Read the model definition and answer for the solid it produces. Units are mm, in the model's axes. A direction names the side the tool comes from. Give positions to 0.01 mm unless a question says otherwise; leave off trailing zeros. Order: outer loops, then holes, each group sorted by start corner. A loop starts at its lowest first (then second) coordinate and runs counter-clockwise, first axis right, second up. Notation, with made-up numbers: (2.5, 53.25) - (57.5, 53.25) arc R27 ccw to (57.5, 85.25) - close; hole circle Ø9 at (47.5, -33). An arc over 180 degrees is marked (long way). Write item = value, one per line.
```python
from build123d import *

# Parameters (mm, degrees)
CORTE_EXTRUS_O1_DEPTH = 3
ESBO_O4_R             = 5
CORTE_EXTRUS_O2_DEPTH = 72.529714105
CHANFRO1_SIZE         = 2
CHANFRO2_SIZE         = 2
CHANFRO3_SIZE         = 1


with BuildPart() as part:
    # Esboço1 → Revolução1 (revolve)
    with BuildSketch(Plane.XY, mode=Mode.PRIVATE) as revolu_o1_sk:
        Polygon((44.5, 0), (44.5, 8), (36.3, 8), (36.3, 18.5), (33.7, 18.5), (33.7, 22), (36.3, 22), (36.3, 27), (33.7, 27), (33.7, 30.5), (36.3, 30.5), (36.3, 35.5), (33.7, 35.5), (33.7, 39), (36.3, 39), (36.3, 46), (24, 46), (24, 12), (0, 12), (0, 0), align=None)
    revolve(revolu_o1_sk.sketch.rotate(Axis((0, 0, 0), (0, 1, 0)), 90), axis=Axis((0, 0, 0), (0, 1, 0)))

    # Esboço2 → Corte-extrusão1 (cut)
    with BuildSketch(Plane(origin=(0, 8, 0), x_dir=(1, 0, 0), z_dir=(0, 1, 0))):
        with BuildLine():
            Line((-5, 43.5), (-5, 45.5))
            ThreePointArc((-5, 45.5), (0, 50.5), (5, 45.5))
            Line((5, 45.5), (5, 43.5))
            ThreePointArc((5, 43.5), (0, 38.5), (-5, 43.5))
        make_face()
        with BuildLine():
            Line((-5, -43.5), (-5, -45.5))
            ThreePointArc((-5, -45.5), (0, -50.5), (5, -45.5))
            Line((5, -45.5), (5, -43.5))
            ThreePointArc((5, -43.5), (0, -38.5), (-5, -43.5))
        make_face()
    extrude(amount=-CORTE_EXTRUS_O1_DEPTH, mode=Mode.SUBTRACT)

    # Esboço4 → Corte-extrusão2 (cut, through all)
    with BuildSketch(Plane(origin=(0, 12, 0), x_dir=(1, 0, 0), z_dir=(0, 1, 0))):
        with Locations(Location((-9.941125497, 9.941125497, 0), (0, 0, 270))):
            Circle(ESBO_O4_R)
        with Locations(Location((9.941125497, 9.941125497, 0), (0, 0, 270))):
            Circle(ESBO_O4_R)
        with Locations(Location((-9.941125497, -9.941125497, 0), (0, 0, 270))):
            Circle(ESBO_O4_R)
        with Locations(Location((9.941125497, -9.941125497, 0), (0, 0, 270))):
            Circle(ESBO_O4_R)
    extrude(amount=-CORTE_EXTRUS_O2_DEPTH, mode=Mode.SUBTRACT)

    # Chanfro1
    chanfro1_edges = [part.edges().sort_by_distance(p)[0] for p in [
        (0, 46, 36.3),
    ]]
    chamfer(chanfro1_edges, length=CHANFRO1_SIZE)

    # Chanfro2
    chanfro2_edges = [part.edges().sort_by_distance(p)[0] for p in [
        (0, 12, 24),
    ]]
    chamfer(chanfro2_edges, length=CHANFRO2_SIZE)

    # Chanfro3
    chanfro3_edges = [part.edges().sort_by_distance(p)[0] for p in [
        (0, 0, 44.5),
    ]]
    chamfer(chanfro3_edges, length=CHANFRO3_SIZE)


solid = part.part
```
1. Flat-ended cylindrical pins translate along their axes: pin 1 (4 mm diameter, centred on y = 19.5, z = -8, fed in from -X); pin 2 (8 mm diameter, centred on x = -26.5, y = 31.5, fed in from -Z); pin 3 (3 mm diameter, centred on x = -13.5, y = 14, fed in from -Z); pin 4 (8 mm diameter, centred on x = 9.94, z = -9.94, fed in from -Y). Find the tip coordinate at first contact, or state that the pin passes through.
Recorded:
pin_1 = -35.75
pin_2 = -28.49
pin_3 = -34.26
pin_4 = through
2. Section B-B (x = -13.5) is taken. Count the separate pieces of the cut face and the enclosed holes in it, and give its area (3 significant figures).
Recorded:
separate_pieces = 3
enclosed_holes = 0
area = 1,660 mm^2
3. Determine the mould class of faces 4 (the face through (14.157, 6.084, 12.629)), 5 (the face through (24, 22, 24)), 6 (the face through (33, 8, -16)), 7 (the face through (24, 39, 24)) for opening direction Y: +Y half, -Y half, draft (parallel to the pull), parting line (faces both ways), or undercut.
Recorded:
face_4 = draft
face_5 = undercut
face_6 = +Y half
face_7 = undercut
4. Straight lines are drawn through the part: L1, parallel to Z at x = -6, y = 2; L2, parallel to X at y = 5, z = -10; L3, parallel to Z at x = -9, y = 2.5. For each, find the intervals that lie inside material, in ascending order. Write a range as [from, to].
Recorded:
L1 = [-44.09, -13.02], [-6.86, 6.86], [13.02, 44.09]
L2 = [-43.36, -14.94], [-4.94, 4.94], [14.94, 43.36]
L3 = [-43.58, -14.85], [-5.03, 5.03], [14.85, 43.58]
5. For faces 1 (the face through (0, 5, -42)), 2 (the face through (-33.413, 20.274, 4.387)), 3 (the face through (22.088, 41.535, 28.806)), determine the directions among +Z, -Z, +X, -X, +Y, -Y from which every point of the face is accessible in a straight line to the end or side of a thin tool.
Recorded:
face_1 = -Z, +Y
face_2 = none
face_3 = +Y
6. Section A-A (y = 10) is taken. Determine the outline of the cut face in (x, z).
Recorded:
outline = circle Ø72.6 at (0, 0); hole circle Ø10 at (-9.94, -9.94); hole circle Ø10 at (-9.94, 9.94); hole circle Ø10 at (9.94, -9.94); hole circle Ø10 at (9.94, 9.94)
